Part model, mm, in its own coordinate system. Coordinates: 2 decimals unless noted, no trailing zeros. Loops run counter-clockwise (first coordinate to the right, second up) from the corner with the lowest first, then second, coordinate; pieces in that order, holes last. Notation, with made-up numbers: M -39,56 L 3,56 A17 cw 3,62 Z; hole C -1.5,56.5 d2. An arc over 180 degrees is marked long. Use a Markdown table: item, result. Add a question column.
1) Band-saw the part on D-D (y = 21.65). List the corners of the cut face in (x, z), plus the area to 3 significant figures.
2) Wall check: probe 1 along Y at (x, z) = (4, -15); probe 2 along Y at (x, z) = (115.7, -42.4); probe 3 along Y at (x, z) = (53.3, -43.6). Give the ranges that are in metal, low to high. Write a range as from..to.
3) Band-saw the part on C-C (x = 53.3). List the corners of the cut face in (y, z).
4) Band-saw the part on A-A (y = 30). List the corners of the cut face in (x, z), plus the area to 3 significant figures.
5) Band-saw the part on B-B (x = 68). List the corners of the cut face in (y, z), plus the area to 3 significant figures.
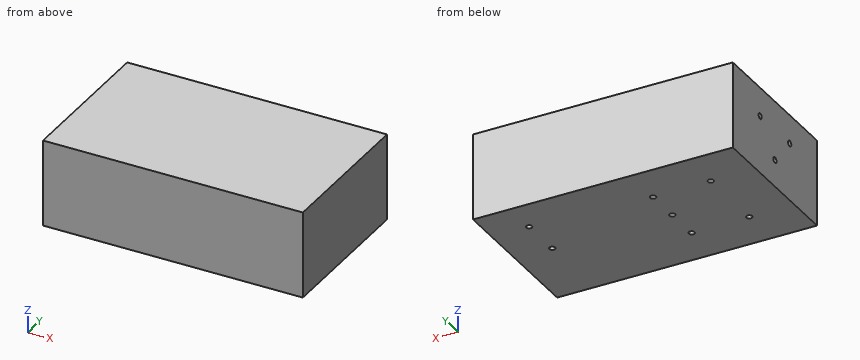
from build123d import *

# Parameters (mm, degrees)
SKETCH1_W           = 135
SKETCH1_H           = 80
BOSS_EXTRUDE1_DEPTH = 45
SKETCH2_R           = 1.5
CUT_EXTRUDE1_DEPTH  = 10
SKETCH3_R           = 1.5
CUT_EXTRUDE2_DEPTH  = 10
CAVITY1_START       = 6.25125
CAVITY1_DEPTH       = 67.4975
CAVITY1_START_2     = 5
CAVITY1_2_DEPTH     = 125


with BuildPart() as part:
    # Sketch1 → Boss-Extrude1 (new body)
    with BuildSketch(Plane.XY):
        with Locations((67.5, 40)):
            Rectangle(SKETCH1_W, SKETCH1_H)
    extrude(amount=-BOSS_EXTRUDE1_DEPTH)

    # Sketch2 → Cut-Extrude1 (cut)
    with BuildSketch(Plane(origin=(0, 0, -45), x_dir=(-1, 0, 0), z_dir=(0, 0, -1))):
        with Locations((-53.3, 40)):
            Circle(SKETCH2_R)
        with Locations((-53.3, 58.35)):
            Circle(SKETCH2_R)
        with Locations((-53.3, 21.65)):
            Circle(SKETCH2_R)
        with Locations((-23.3, 58.35)):
            Circle(SKETCH2_R)
        with Locations((-23.3, 21.65)):
            Circle(SKETCH2_R)
        with Locations((-115.7, 40)):
            Circle(SKETCH2_R)
        with Locations((-115.7, 62)):
            Circle(SKETCH2_R)
    extrude(amount=-CUT_EXTRUDE1_DEPTH, mode=Mode.SUBTRACT)

    # Sketch3 → Cut-Extrude2 (cut)
    with BuildSketch(Plane.ZY):
        with Locations((-15, 54.05)):
            Circle(SKETCH3_R)
        with Locations((-15, 25.95)):
            Circle(SKETCH3_R)
        with Locations((-31, 40)):
            Circle(SKETCH3_R)
    extrude(amount=-CUT_EXTRUDE2_DEPTH, mode=Mode.SUBTRACT)

    # Cavity1: read off the stored shape, not the designer's step
    # Cavity1 outline → Cavity1 (cut)
    with BuildSketch(Plane(origin=(0, 0, 0), x_dir=(1, 0, 0), z_dir=(0, 1, 0)).offset(CAVITY1_START)):
        Polygon((127.780327673, 40.35), (7.219672327, 40.35), (6.294, 5), (128.706, 5), align=None)
    extrude(amount=CAVITY1_DEPTH, mode=Mode.SUBTRACT)

    # Cavity1 2 outline → Cavity1 2 (add)
    with BuildSketch(Plane.YZ.offset(CAVITY1_START_2)):
        Polygon((73.74875, -5), (72.818495136, -40.35), (73.74875, -40.35), align=None)
        Polygon((7.181504864, -40.35), (6.25125, -5), (6.25125, -40.35), align=None)
    extrude(amount=CAVITY1_2_DEPTH)


solid = part.part
Entries:
| question | item | result |
|---|---|---|
| 1 | outline | M 0,-45 L 21.8,-45 L 21.8,-40.35 L 7.22,-40.35 L 6.29,-5 L 128.71,-5 L 127.78,-40.35 L 54.8,-40.35 L 54.8,-45 L 135,-45 L 135,0 L 0,0 Z; M 24.8,-45 L 51.8,-45 L 51.8,-40.35 L 24.8,-40.35 Z |
| 1 | area | 1,750 mm2 |
| 2 | probe 1 | 0..24.45, 27.45..52.55, 55.55..80 |
| 2 | probe 2 | 0..38.5, 41.5..60.5, 63.5..80 |
| 2 | probe 3 | 0..20.15, 23.15..38.5, 41.5..56.85, 59.85..80 |
| 3 | outline | M 0,-45 L 20.15,-45 L 20.15,-40.35 L 7.18,-40.35 L 6.25,-5 L 73.75,-5 L 72.82,-40.35 L 59.85,-40.35 L 59.85,-45 L 80,-45 L 80,0 L 0,0 Z; M 23.15,-45 L 38.5,-45 L 38.5,-40.35 L 23.15,-40.35 Z; M 41.5,-45 L 56.85,-45 L 56.85,-40.35 L 41.5,-40.35 Z |
| 4 | outline | M 0,-45 L 135,-45 L 135,0 L 0,0 Z; hole M 6.29,-5 L 7.22,-40.35 L 127.78,-40.35 L 128.71,-5 Z |
| 4 | area | 1,780 mm2 |
| 5 | outline | M 0,-45 L 80,-45 L 80,0 L 0,0 Z; hole M 6.25,-5 L 7.18,-40.35 L 72.82,-40.35 L 73.75,-5 Z |
| 5 | area | 1,250 mm2 |
